Work out the finished part from the listing and answer in its coordinate system (mm). A direction names the side the tool comes from. Give positions to 0.01 mm unless a question says otherwise; leave off trailing zeros. Loops run counter-clockwise (first coordinate to the right, second up) from the corner with the lowest first, then second, coordinate; pieces in that order, holes last. Notation, with made-up numbers: M -12,66 L 16,66 A29 ccw 16,87 Z; hole C 32,-16 d1. An arc over 180 degrees is marked long. Answer in a Markdown table with one row per item. Add a question column.
Autodesk Inventor part; units mm, degrees
ref_plane "YZ Plane" through (0, 0, 0) normal (1, 0, 0) x (0, 1, 0)
ref_plane "XZ Plane" through (0, 0, 0) normal (0, 1, 0) x (-1, 0, 0)
ref_plane "XY Plane" through (0, 0, 0) normal (0, 0, 1) x (1, 0, 0)
sketch "Sketch1" plane through (0, 0, 0) normal (0, 0, 1) x (1, 0, 0)
  line L0 (0, 0) -> (14.5304, 0)
  line L1 (-8.7854, 6.6412) -> (8.2146, 6.6412)
  line L2 (8.2146, 1.6412) -> (2.0946, 1.6412)
  line L3 (2.0946, 1.6412) -> (2.0946, -0.3588)
  line L4 (2.0946, -0.3588) -> (5.4596, -0.3588)
  line L5 (2.5721, -3.1588) -> (-3.1429, -3.1588)
  line L6 (-3.1429, -3.1588) -> (-6.0304, -1.1208)
  line L7 (-6.0304, -1.1208) -> (-6.0304, -0.3588)
  line L8 (-6.0304, -0.3588) -> (-2.6654, -0.3588)
  line L9 (-2.6654, -0.3588) -> (-2.6654, 1.6412)
  line L10 (-2.6654, 1.6412) -> (-8.7854, 1.6412)
  line L11 (-8.7854, 1.6412) -> (-8.7854, 6.6412)
  line L12 (5.4596, -0.3588) -> (5.4596, -1.1208)
  line L13 (5.4596, -1.1208) -> (2.5721, -3.1588)
  line L14 (8.2146, 6.6412) -> (28.1746, 6.6412)
  line L15 (28.1746, 6.6412) -> (28.1746, 1.6412)
  line L16 (28.1746, 1.6412) -> (8.2146, 1.6412)
  dimension "d2" = 5
  dimension "d3" = 2
  dimension "d4" = 4.76
  dimension "d6" = 11.49
  dimension "d7" = 2.755
  dimension "d8" = 5.715
  dimension "d9" = 5.6425
  dimension "d10" = 6.12
  dimension "d11" = 0.762
  dimension "d12" = 0.762
  dimension "d16" = 26.08
  dimension "d50" = 144.786
  dimension "d51" = 2.8875
extrude "Extrusion1" add sketch "Sketch1" along normal blind 19.05
sketch "Sketch3" plane through (-8.7854, 6.6412, 0) normal (0, 1, 0) x (1, 0, 0)
  line L0 (36.96, 0) -> (36.96, -19.05)
  line L1 (0, 0) -> (36.96, 0)
  line L2 (36.96, -19.05) -> (0, -19.05)
  point P0 (8.7854, 0)
  point P1 (31.88, -15.875)
  point P2 (31.88, -3.175)
  dimension "d27" = 5.08
  dimension "d28" = 5.08
  dimension "d36" = 3.175
  dimension "d37" = 3.175
hole "Hole1" at (23.0946, 6.6412, 15.875) at (23.0946, 6.6412, 3.175) direction (0, -1, 0) diameter 4.064 depth 25.4 tip angle 118
equation "\"d7\" = -0.5 * d6 + 0.5 * d0"
equation "\"d9\" = -0.5 * d8 + 0.5 * d0"
equation "\"d10\" = -0.5 * d4 + 0.5 * d0"
equation "\"d12\" = d11"
properties part number "Sliderfor2020"
(1) The mould has two halves that part along Y. Classify faces 1 (the face through (9, 6.641, 9)), 2 (the face through (0, -3.159, 9)), 3 (the face through (28.175, 4, 9)), 4 (the face through (2.095, 1, 9)): pulls with the +Y half, pulls with the -Y half, needs draft (parallel to the pull), parting line crosses it, or undercut.
(2) Consider line 1 along Y through (x, z) = (18, 3); line 2 along X through (y, z) = (-0.5, 15.5); line 3 along Y through (x, z) = (5, 12.5). Determine where each line is inside the solid, lowest interval first. Write a range as from..to.
(3) Each of these flat-tipped pins is pushed along its axis until it touches: P1, Ø0.6, axis at y = 1, z = 12, coming from the -X side; P2, Ø4, axis at y = -1.5, z = 5, coming from the +X side; P3, Ø0.6, axis at y = 1, z = 11, coming from the +X side; P4, Ø3.5, axis at x = 23.09, z = 3.18, coming from the -Y side. Where does it stop, or does it pass through?
(4) Section D-D, the plane y = 3 is taken. Determine the outline of the cut face in (x, z) (3 decimals).
(5) Section C-C, the plane z = 6.25 is taken. Determine the outline of the cut face in (x, y), and give its area (3 significant figures).
(6) Which of the six approach directions +Z, -Z, +X, -X, +Y, -Y give full straight-line access (tool end or side, diameter ignored) to faces 5 (the face through (4, -0.359, 9)), 6 (the face through (-6, 1.641, 9)), 7 (the face through (25.078, 4.106, 2.735))?
(7) Section A-A, the plane z = 2 is taken. Determine the outline of the cut face in (x, y), and give its area (3 significant figures).
(8) Section B-B, the plane x = -5 is taken. Determine the outline of the cut face in (y, z).
Numbers:
| question | item | result |
|---|---|---|
| 1 | face 1 | pulls with the +Y half |
| 1 | face 2 | pulls with the -Y half |
| 1 | face 3 | needs draft |
| 1 | face 4 | undercut |
| 2 | line 1 | y = 1.64..6.64 |
| 2 | line 2 | x = -6.03..5.46 |
| 2 | line 3 | y = -1.45..-0.36, 1.64..6.64 |
| 3 | P1 | stops at x = -2.67 |
| 3 | P2 | stops at x = 5.46 |
| 3 | P3 | stops at x = 2.09 |
| 3 | P4 | passes through |
| 4 | outline | M -8.785,0 L 28.175,0 L 28.175,19.05 L -8.785,19.05 Z; hole C 23.095,3.175 d4.064; hole C 23.095,15.875 d4.064 |
| 5 | outline | M -8.79,1.64 L -2.67,1.64 L -2.67,-0.36 L -6.03,-0.36 L -6.03,-1.12 L -3.14,-3.16 L 2.57,-3.16 L 5.46,-1.12 L 5.46,-0.36 L 2.09,-0.36 L 2.09,1.64 L 28.17,1.64 L 28.17,6.64 L -8.79,6.64 Z |
| 5 | area | 221 mm² |
| 6 | face 5 | +Z, -Z, +X |
| 6 | face 6 | +Z, -Z, -X |
| 6 | face 7 | +Y, -Y |
| 7 | outline | M -8.79,1.64 L -2.67,1.64 L -2.67,-0.36 L -6.03,-0.36 L -6.03,-1.12 L -3.14,-3.16 L 2.57,-3.16 L 5.46,-1.12 L 5.46,-0.36 L 2.09,-0.36 L 2.09,1.64 L 21.44,1.64 L 21.44,6.64 L -8.79,6.64 Z; M 24.75,1.64 L 28.17,1.64 L 28.17,6.64 L 24.75,6.64 Z |
| 7 | area | 204 mm² |
| 8 | outline | M -1.85,0 L -0.36,0 L -0.36,19.05 L -1.85,19.05 Z; M 1.64,0 L 6.64,0 L 6.64,19.05 L 1.64,19.05 Z |
